Part model, mm, in its own coordinate system. Face numbers are marked on the shaded views. A direction names the side the tool comes from. Give positions to 0.01 mm unless a question says otherwise; leave off trailing zeros. Write each loop counter-clockwise with the first axis right and the second up, starting at its lowest first coordinate (ties: lowest second). Pieces come first, ordered by that corner, then holes. Notation, with made-up numbers: M -30.5,83.25 L 15.5,83.25 A24 cw 15.5,108.25 Z; hole C 65,-11 d2. An arc over 180 degrees is marked long. Use a Markdown table: item, result.
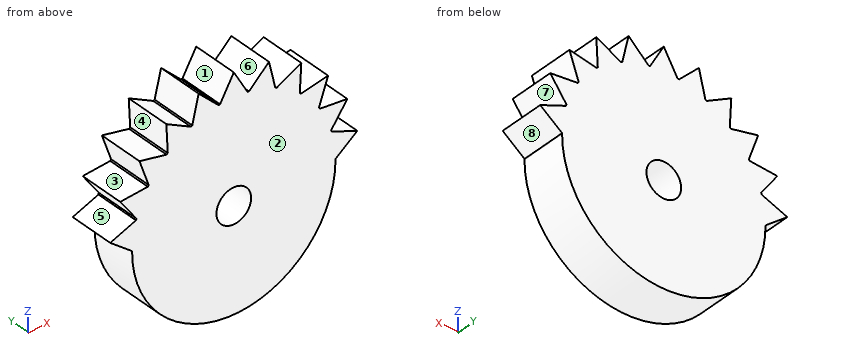
```python
from build123d import *

# Parameters (mm, degrees)
F1_DEPTH = 12.7
F2_R     = 4.7625
F3_DEPTH = 12.7


with BuildPart() as f1:
    # F0 (on Front) → F1 (new body)
    with BuildSketch(Plane.XZ):
        with BuildLine():
            ThreePointArc((26.865064, 7.665134), (27.652819, 3.975875), (27.936358, 0.214121))
            Line((27.936358, 0.214121), (33.938185, 4.879574))
            Line((33.938185, 4.879574), (26.865064, 7.665134))
        make_face()
        with BuildLine():
            ThreePointArc((23.617322, 14.923406), (25.412552, 11.605523), (26.744415, 8.076029))
            Line((26.744415, 8.076029), (31.188715, 14.243409))
            Line((31.188715, 14.243409), (23.617322, 14.923406))
        make_face()
        with BuildLine():
            ThreePointArc((18.456246, 20.972672), (21.113511, 18.294961), (23.385798, 15.283665))
            Line((23.385798, 15.283665), (25.912521, 22.453327))
            Line((25.912521, 22.453327), (18.456246, 20.972672))
        make_face()
        with BuildLine():
            ThreePointArc((11.799954, 25.322856), (15.103979, 23.50225), (18.132602, 21.25311))
            Line((18.132602, 21.25311), (18.537048, 28.84421))
            Line((18.537048, 28.84421), (11.799954, 25.322856))
        make_face()
        with BuildLine():
            ThreePointArc((-27.936358, 0.214121), (-0.107061, -27.936974), (27.937179, 0))
            ThreePointArc((27.937179, 0), (27.936974, 0.107061), (27.936358, 0.214121))
            ThreePointArc((27.936358, 0.214121), (27.652819, 3.975875), (26.865064, 7.665134))
            ThreePointArc((26.865064, 7.665134), (26.805527, 7.870813), (26.744415, 8.076029))
            ThreePointArc((26.744415, 8.076029), (25.412552, 11.605523), (23.617322, 14.923406))
            ThreePointArc((23.617322, 14.923406), (23.50225, 15.103979), (23.385798, 15.283665))
            ThreePointArc((23.385798, 15.283665), (21.113511, 18.294961), (18.456246, 20.972672))
            ThreePointArc((18.456246, 20.972672), (18.294961, 21.113511), (18.132602, 21.25311))
            ThreePointArc((18.132602, 21.25311), (15.103979, 23.50225), (11.799954, 25.322856))
            ThreePointArc((11.799954, 25.322856), (11.605523, 25.412552), (11.410412, 25.500754))
            ThreePointArc((11.410412, 25.500754), (7.870813, 26.805527), (4.187699, 27.621534))
            ThreePointArc((4.187699, 27.621534), (3.975875, 27.652819), (3.763817, 27.682479))
            ThreePointArc((3.763817, 27.682479), (0, 27.937179), (-3.763817, 27.682479))
            ThreePointArc((-3.763817, 27.682479), (-3.975875, 27.652819), (-4.187699, 27.621534))
            ThreePointArc((-4.187699, 27.621534), (-7.870813, 26.805527), (-11.410412, 25.500754))
            ThreePointArc((-11.410412, 25.500754), (-11.605523, 25.412552), (-11.799954, 25.322856))
            ThreePointArc((-11.799954, 25.322856), (-15.103979, 23.50225), (-18.132602, 21.25311))
            ThreePointArc((-18.132602, 21.25311), (-18.294961, 21.113511), (-18.456246, 20.972672))
            ThreePointArc((-18.456246, 20.972672), (-21.113511, 18.294961), (-23.385798, 15.283665))
            ThreePointArc((-23.385798, 15.283665), (-23.50225, 15.103979), (-23.617322, 14.923406))
            ThreePointArc((-23.617322, 14.923406), (-25.412552, 11.605523), (-26.744415, 8.076029))
            ThreePointArc((-26.744415, 8.076029), (-26.805527, 7.870813), (-26.865064, 7.665134))
            ThreePointArc((-26.865064, 7.665134), (-27.652819, 3.975875), (-27.936358, 0.214121))
        make_face()
        with BuildLine():
            ThreePointArc((4.187699, 27.621534), (7.870813, 26.805527), (11.410412, 25.500754))
            Line((11.410412, 25.500754), (9.659815, 32.898307))
            Line((9.659815, 32.898307), (4.187699, 27.621534))
        make_face()
        with BuildLine():
            ThreePointArc((-3.763817, 27.682479), (0, 27.937179), (3.763817, 27.682479))
            Line((3.763817, 27.682479), (0, 34.287179))
            Line((0, 34.287179), (-3.763817, 27.682479))
        make_face()
        with BuildLine():
            Line((-9.659815, 32.898307), (-11.410412, 25.500754))
            ThreePointArc((-11.410412, 25.500754), (-7.870813, 26.805527), (-4.187699, 27.621534))
            Line((-4.187699, 27.621534), (-9.659815, 32.898307))
        make_face()
        with BuildLine():
            Line((-18.537048, 28.84421), (-18.132602, 21.25311))
            ThreePointArc((-18.132602, 21.25311), (-15.103979, 23.50225), (-11.799954, 25.322856))
            Line((-11.799954, 25.322856), (-18.537048, 28.84421))
        make_face()
        with BuildLine():
            Line((-25.912521, 22.453327), (-23.385798, 15.283665))
            ThreePointArc((-23.385798, 15.283665), (-21.113511, 18.294961), (-18.456246, 20.972672))
            Line((-18.456246, 20.972672), (-25.912521, 22.453327))
        make_face()
        with BuildLine():
            Line((-31.188715, 14.243409), (-26.744415, 8.076029))
            ThreePointArc((-26.744415, 8.076029), (-25.412552, 11.605523), (-23.617322, 14.923406))
            Line((-23.617322, 14.923406), (-31.188715, 14.243409))
        make_face()
        with BuildLine():
            Line((-33.938185, 4.879574), (-27.936358, 0.214121))
            ThreePointArc((-27.936358, 0.214121), (-27.652819, 3.975875), (-26.865064, 7.665134))
            Line((-26.865064, 7.665134), (-33.938185, 4.879574))
        make_face()
    extrude(amount=F1_DEPTH)

    # F2 (on face) → F3 (cut)
    with BuildSketch(Plane.XZ):
        Circle(F2_R)
    extrude(amount=F3_DEPTH, mode=Mode.SUBTRACT)


solid = f1.part
```
1. Drop flat-ended pins along their axis: P1, Ø2, axis at y = -8.5, z = -15.5, coming from the +X side; P2, Ø2, axis at x = 13.5, y = -3, coming from the +Z side; P3, Ø4, axis at x = 8.5, y = -5.5, coming from the +Z side. Give the stop position or say it passes through.
Findings below:
| item | result |
|---|---|
| P1 | x = 23.88 |
| P2 | z = 26.73 |
| P3 | z = 32.9 |
2. Drill centre lines: L1, parallel to X at y = -10.5, z = -2.5; L2, parallel to Z at x = -29.5, y = -9; L3, parallel to Z at x = -2.5, y = -1.5. Where is each one in solid material? Low to high.
Findings below:
| item | result |
|---|---|
| L1 | -27.83 to -4.05, 4.05 to 27.83 |
| L2 | 1.43 to 6.63, 11.9 to 14.4 |
| L3 | -27.83 to -4.05, 4.05 to 29.9 |
3. Cut at A-A, the plane x = -3. Give the cut face in (y, z).
Findings below:
| item | result |
|---|---|
| outline | M -12.7,-27.78 L 0,-27.78 L 0,-3.7 L -12.7,-3.7 Z; M -12.7,3.7 L 0,3.7 L 0,29.02 L -12.7,29.02 Z |
4. Tool access for the marked faces 5, 6, 7 and 8: list every direction of +Z, -Z, +X, -X, +Y, -Y with a clear straight run to the whole face (end or side of a thin tool).
Findings below:
| item | result |
|---|---|
| face 5 | -X, +Y, -Y |
| face 6 | +Z, +Y, -Y |
| face 7 | +X, +Y, -Y |
| face 8 | -Z, +X, +Y, -Y |
5. Cut at B-B, the plane x = 7. Give the cut face in (y, z).
Findings below:
| item | result |
|---|---|
| outline | M -12.7,-27.05 L 0,-27.05 L 0,30.33 L -12.7,30.33 Z |
6. Two-plate mould, pull along Z, no slides. Class the marked faces 1, 2, 3 and 4: released by +Z, released by -Z, zero draft, split by the parting line, or undercut.
Findings below:
| item | result |
|---|---|
| face 1 | released by +Z |
| face 2 | zero draft |
| face 3 | undercut |
| face 4 | undercut |
7. Cut at C-C, the plane x = -17. Give the cut face in (y, z).
Findings below:
| item | result |
|---|---|
| outline | M -12.7,-22.17 L 0,-22.17 L 0,28.04 L -12.7,28.04 Z |
